Source: CAD feature listing. Evaluate the final solid. Frame: model axes, mm. Face numbers are marked on the shaded views. Coordinates: 2 decimals unless noted, no trailing zeros. Order: outer loops, then holes, each group sorted by start corner. A loop starts at its lowest first (then second) coordinate and runs counter-clockwise, first axis right, second up.
Item 1: Section B-B on x = 28. Return the cut outline in (y, z).
Item 2: Mould query, pull axis X, two halves, no side actions, for the marked faces 1, 2, 3 and 4. Classes: released by +X, released by -X, zero draft, split by the parting line, or undercut.
Item 3: Section C-C on z = 10. Return the cut outline in (x, y), then the cut area to 3 significant figures.
Item 4: Contact query for a flat-ended pin moving along its axis: P1, Ø12, axis at x = 22, z = 22.5, coming from the +Y side. Output: stop coordinate, or through.
Item 5: Section A-A on y = 7.25. Return the cut outline in (x, z), then the cut area to 3 significant figures.
Item 6: Ray query, line 1 (Z direction, x = 34, y = 6); line 2 (X direction, y = 3.75, z = 23); line 3 (X direction, y = 5.25, z = -1). Return the intervals inside material, ascending.
from build123d import *

# Parameters (mm, degrees)
SKETCH1_W           = 93.218
SKETCH1_H           = 86.868
BOSS_EXTRUDE1_DEPTH = 10.16
SKETCH2_W           = 90.424
SKETCH2_H           = 84.074
CUT_EXTRUDE1_DEPTH  = 5.842
SKETCH3_W           = 84.582
SKETCH3_H           = 78.232
CUT_EXTRUDE2_DEPTH  = 2.286
FILLET1_R           = 10.16


with BuildPart() as part:
    # Sketch1 → Boss-Extrude1 (new body)
    with BuildSketch(Plane(origin=(0, 0, 0), x_dir=(1, 0, 0), z_dir=(0, 1, 0))):
        Rectangle(SKETCH1_W, SKETCH1_H)
    extrude(amount=BOSS_EXTRUDE1_DEPTH)

    # Sketch2 → Cut-Extrude1 (cut)
    with BuildSketch(Plane(origin=(0, 10.16, 0), x_dir=(1, 0, 0), z_dir=(0, 1, 0))):
        Rectangle(SKETCH2_W, SKETCH2_H)
    extrude(amount=-CUT_EXTRUDE1_DEPTH, mode=Mode.SUBTRACT)

    # Sketch3 → Cut-Extrude2 (cut)
    with BuildSketch(Plane(origin=(0, 4.318, 0), x_dir=(1, 0, 0), z_dir=(0, 1, 0))):
        Rectangle(SKETCH3_W, SKETCH3_H)
    extrude(amount=-CUT_EXTRUDE2_DEPTH, mode=Mode.SUBTRACT)

    # Fillet1
    fillet1_edges = [part.edges().sort_by_distance(p)[0] for p in [
        (45.212, 7.239, -42.037),
        (45.212, 7.239, 42.037),
        (-45.212, 7.239, 42.037),
        (-45.212, 7.239, -42.037),
        (42.291, 3.175, -39.116),
        (42.291, 3.175, 39.116),
        (-42.291, 3.175, 39.116),
        (-42.291, 3.175, -39.116),
        (46.609, 5.08, 43.434),
        (-46.609, 5.08, 43.434),
        (-46.609, 5.08, -43.434),
        (46.609, 5.08, -43.434),
    ]]
    fillet(fillet1_edges, radius=FILLET1_R)


solid = part.part
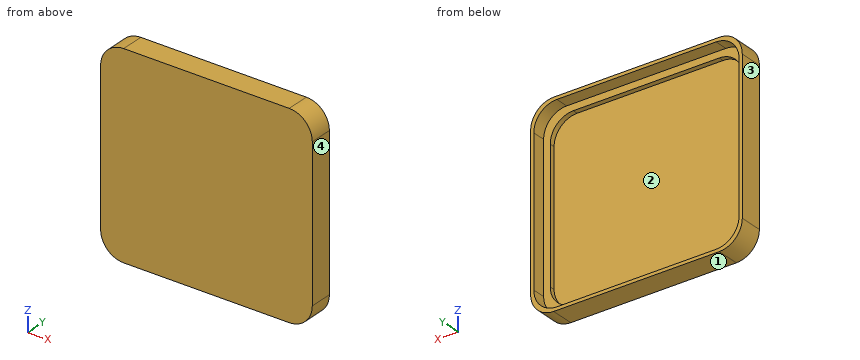
Answer list:
1. outline: (0, -43.43) - (10.16, -43.43) - (10.16, -42.04) - (4.32, -42.04) - (4.32, -39.12) - (2.03, -39.12) - (2.03, 39.12) - (4.32, 39.12) - (4.32, 42.04) - (10.16, 42.04) - (10.16, 43.43) - (0, 43.43) - close
2. face 1: zero draft
2. face 2: undercut
2. face 3: released by -X
2. face 4: released by +X
3. outline: (-46.61, 0) - (46.61, 0) - (46.61, 10.16) - (45.21, 10.16) - (45.21, 4.32) - (42.29, 4.32) - (42.29, 2.03) - (-42.29, 2.03) - (-42.29, 4.32) - (-45.21, 4.32) - (-45.21, 10.16) - (-46.61, 10.16) - close
3. area: 225 mm2
4. P1: stops at y = 2.03
5. outline: (-46.61, -33.27) arc R10.16 ccw to (-36.45, -43.43) - (36.45, -43.43) arc R10.16 ccw to (46.61, -33.27) - (46.61, 33.27) arc R10.16 ccw to (36.45, 43.43) - (-36.45, 43.43) arc R10.16 ccw to (-46.61, 33.27) - close; hole (-45.21, -31.88) arc R10.16 ccw to (-35.05, -42.04) - (35.05, -42.04) arc R10.16 ccw to (45.21, -31.88) - (45.21, 31.88) arc R10.16 ccw to (35.05, 42.04) - (-35.05, 42.04) arc R10.16 ccw to (-45.21, 31.88) - close
5. area: 495 mm2
6. line 1: z = -43.43 to -42.04, 42.04 to 43.43
6. line 2: x = -46.61 to -42.29, 42.29 to 46.61
6. line 3: x = -46.61 to -45.21, 45.21 to 46.61
